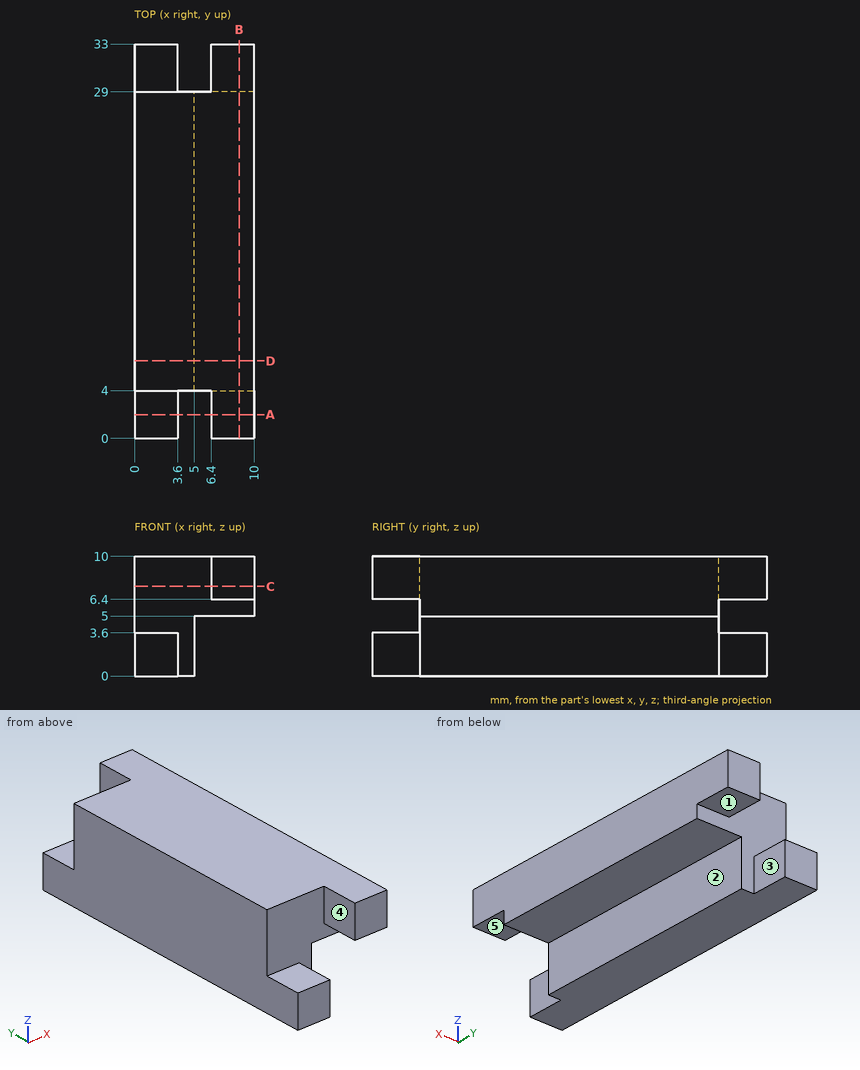
Could you check a few things on this drawing? It's one solid part, dimensions in mm from its lowest x, y, z. A direction names the side the tool comes from. Give positions to 0.01 mm unless a question says otherwise; leave off trailing zeros. Order: outer loops, then holes, each group sorted by start corner. A loop starts at its lowest first (then second) coordinate and runs counter-clockwise, first axis right, second up.
1. Which directions (+Z, -Z, +X, -X, +Y, -Y) give clear straight access to the entire face, cutting with the end or side of a thin tool? Please do the marked faces 1, 2, 3, 4 and 5.
Answers below:
face 1: -Z, +X, -X, +Y
face 2: -Z, +X, +Y, -Y
face 3: +Z, -Z, +X, +Y
face 4: +Z, -Z, -X, -Y
face 5: -Z, +X, -X, -Y
2. Suppose I cut it at B-B (x = 8.75). Write out the boundary of the cut face in (y, z).
Answers below:
outline: (0, 6.4) - (4, 6.4) - (4, 5) - (29, 5) - (29, 6.4) - (33, 6.4) - (33, 10) - (0, 10) - close
3. Suppose I cut it at D-D (y = 6.5). Write out the boundary of the cut face in (x, z), plus the area to 3 significant figures.
Answers below:
outline: (0, 0) - (5, 0) - (5, 5) - (10, 5) - (10, 10) - (0, 10) - close
area: 75.0 mm2
4. For pin 1 (5 mm diameter, centred on x = 4, z = 3.5, fed in from -Y); pin 2 (1.1 mm diameter, centred on y = 30.5, z = 7.5, fed in from -X); pin 3 (1.1 mm diameter, centred on x = 8, y = 2.5, fed in from -Z); pin 4 (1.1 mm diameter, centred on y = 1.5, z = 1, fed in from +X), each with a flat end and sliding along its axis, tell me the tip position at first contact or that it passes through.
Answers below:
pin 1: stops at y = 0
pin 2: stops at x = 6.4
pin 3: stops at z = 6.4
pin 4: stops at x = 3.6
5. Suppose I cut it at C-C (z = 7.5). Write out the boundary of the cut face in (x, y).
Answers below:
outline: (0, 4) - (6.4, 4) - (6.4, 0) - (10, 0) - (10, 33) - (6.4, 33) - (6.4, 29) - (0, 29) - close
6. Suppose I cut it at A-A (y = 2). Write out the boundary of the cut face in (x, z), plus the area to 3 significant figures.
Answers below:
outline: (0, 0) - (3.6, 0) - (3.6, 3.6) - (0, 3.6) - close; (6.4, 6.4) - (10, 6.4) - (10, 10) - (6.4, 10) - close
area: 25.9 mm2
7. I need wall thicknesses on L1, parallel to Z at x = 0.5, y = 31; L2, parallel to Z at x = 7.5, y = 9; L3, parallel to Y at x = 5.5, z = 6.5. Which ranges of each line are inside material? Lowest first, please.
Answers below:
L1: z = 0 to 3.6
L2: z = 5 to 10
L3: y = 4 to 29
